Geometry check sheet. Reference: the model listing, model coordinates, mm. Face numbers are marked on the shaded views. A direction names the side the tool comes from. Give positions to 0.01 mm unless a question says otherwise; leave off trailing zeros. Write each loop counter-clockwise with the first axis right and the second up, starting at its lowest first coordinate (ties: lowest second). Pieces come first, ordered by that corner, then holes.
(1) Cross-section at B-B (y = 376.5). Record the boundary of the cut face in (x, z), and give its area (3 significant figures).
(2) Depth check by flat-ended pin: P1, Ø16.5, axis at x = -287.5, y = 656, coming from the +Z side; P2, Ø10, axis at x = -304, y = 526.5, coming from the +Z side. Enter the tip coordinate at first touch or a pass-through.
(3) Cross-section at C-C (z = 182.5). Record the boundary of the cut face in (x, y).
(4) Cross-section at A-A (x = -221.5). Record the boundary of the cut face in (y, z).
(5) Tool access check on the marked faces 1 and 2. Record the directions out of +Z, -Z, +X, -X, +Y, -Y that give a thin tool (end or side, any length) a straight path to the whole face; none if there is none.
(6) Thickness scan on line 1 along Z through (x, y) = (-281, 684); line 2 along X through (y, z) = (628, 42); line 3 along X through (y, z) = (408, 10). Record the ranges inside material, lowest first.
(7) Cross-section at D-D (x = -139.5). Record the boundary of the cut face in (y, z) (3 decimals), and give its area (3 significant figures).
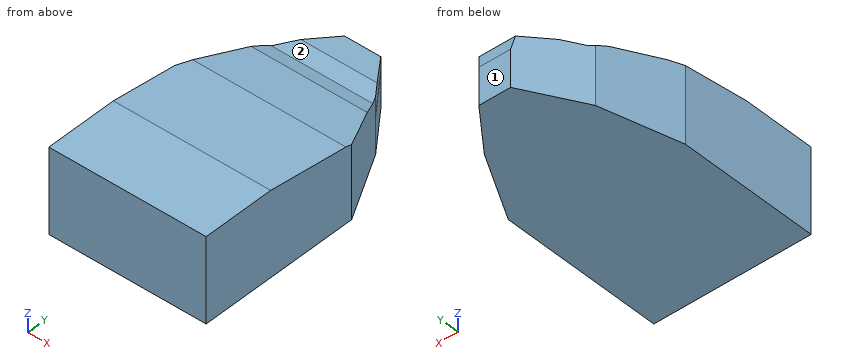
```python
from build123d import *

# Parameters (mm, degrees)
BOSS_EXTRUDE1_DEPTH = 101.6
BOSS_EXTRUDE2_DEPTH = 431.8
CUT_EXTRUDE1_DEPTH  = 132.021743181
CUT_EXTRUDE2_DEPTH  = 132.021743181
SKETCH5_W           = 672.515990181
SKETCH5_H           = 895.069856367
CUT_EXTRUDE3_DEPTH  = 233.621743181


with BuildPart() as part:
    # Sketch1 → Boss-Extrude1 (new body)
    with BuildSketch(Plane.XY):
        Polygon((0, 0), (431.8, 0), (431.8, 387.403361345), (377.065490396, 602.774956458), (285.641844577, 762), (198.504201681, 762), (102.453781513, 637.134453782), (0, 448.235294118), align=None)
    boss_extrude1 = extrude(amount=BOSS_EXTRUDE1_DEPTH)

    # Sketch2 → Boss-Extrude2 (add)
    with BuildSketch(Plane.ZY):
        Polygon((101.6, 0), (232.621743181, 0), (232.621743181, 198.64821401), (204.451845393, 430.506603568), (172.780455352, 570.81191653), (155.089264466, 615.704741573), (155.089264466, 670.908278379), (139.607943989, 752.787376516), (101.6, 762), align=None)
    boss_extrude2 = extrude(amount=-BOSS_EXTRUDE2_DEPTH)

    # Sketch3 → Cut-Extrude1 (cut, through all)
    with BuildSketch(Plane(origin=(0, 0, 101.6), x_dir=(-1, 0, 0), z_dir=(0, 0, -1))):
        Polygon((0, 448.235294118), (-102.079559314, 636.444481603), (-205.052343037, 770.512583763), (-205.052343037, 987.342816442), (227.879484492, 941.92173413), (179.71587047, 482.849418415), align=None)
    cut_extrude1 = extrude(amount=-CUT_EXTRUDE1_DEPTH, mode=Mode.SUBTRACT)

    # Sketch4 → Cut-Extrude2 (cut, through all)
    with BuildSketch(Plane(origin=(0, 0, 101.6), x_dir=(-1, 0, 0), z_dir=(0, 0, -1))):
        Polygon((-431.8, 387.403361345), (-377.065490396, 602.774956458), (-285.641844577, 762), (-386.647779508, 961.526140846), (-935.090979015, 961.526140846), (-884.913915701, 472.949119069), align=None)
    cut_extrude2 = extrude(amount=-CUT_EXTRUDE2_DEPTH, mode=Mode.SUBTRACT)

    # Mirror1: Boss-Extrude1, Boss-Extrude2, Cut-Extrude1, Cut-Extrude2 across plane
    add(boss_extrude1.mirror(Plane(origin=(0, 0, 0), x_dir=(0, 0, 1), z_dir=(1, 0, 0))))
    add(boss_extrude2.mirror(Plane(origin=(0, 0, 0), x_dir=(0, 0, 1), z_dir=(1, 0, 0))))
    add(cut_extrude1.mirror(Plane(origin=(0, 0, 0), x_dir=(0, 0, 1), z_dir=(1, 0, 0))), mode=Mode.SUBTRACT)
    add(cut_extrude2.mirror(Plane(origin=(0, 0, 0), x_dir=(0, 0, 1), z_dir=(1, 0, 0))), mode=Mode.SUBTRACT)

    # Sketch5 → Cut-Extrude3 (cut, through all)
    with BuildSketch(Plane.XY):
        with Locations((336.257995091, 447.534928184)):
            Rectangle(SKETCH5_W, SKETCH5_H)
    extrude(amount=CUT_EXTRUDE3_DEPTH, mode=Mode.SUBTRACT)


solid = part.part
```
Reply:
1. outline: (-431.8, 0) - (0, 0) - (0, 211.01) - (-431.8, 211.01) - close
1. area: 91,100 mm2
2. P1: stops at z = 155.09
2. P2: stops at z = 183.91
3. outline: (-431.8, 0) - (0, 0) - (0, 448.24) - (-43.13, 527.75) - (-396.13, 527.75) - (-431.8, 387.4) - close
4. outline: (0, 0) - (762, 0) - (762, 101.6) - (752.79, 139.61) - (670.91, 155.09) - (615.7, 155.09) - (570.81, 172.78) - (430.51, 204.45) - (198.65, 232.62) - (0, 232.62) - close
5. face 1: +Z, -Z, +X, -X, +Y
5. face 2: +Z, +X, -X, +Y
6. line 1: z = 0 to 152.61
6. line 2: x = -362.58 to -97.5
6. line 3: x = -426.57 to 0
7. outline: (0, 0) - (685.295, 0) - (685.295, 101.6) - (685.165, 101.6) - (685.165, 152.394) - (670.908, 155.089) - (615.705, 155.089) - (570.812, 172.78) - (430.507, 204.452) - (198.648, 232.622) - (0, 232.622) - close
7. area: 141,000 mm2
